The model under review builds one solid part; all positions refer to its coordinate system, in mm. Face numbers are marked on the shaded views. A direction names the side the tool comes from. Coordinates: 2 decimals unless noted, no trailing zeros. Loops run counter-clockwise (first coordinate to the right, second up) from the corner with the lowest first, then second, coordinate; pieces in that order, holes last. Notation, with made-up numbers: M 64,-6.5 L 92,-6.5 A12 cw 92,-1.5 Z; hole C 87.5,-28.75 d7. An arc over 180 degrees is marked long. One line per item, written item: value.
Autodesk Inventor part; units mm, degrees
ref_plane "aa2_XY" through (12.7, 0, 0) normal (0, 1, 0) x (1, 0, 0)
ref_plane "aa2_YZ" through (12.7, 0, 0) normal (1, 0, 0) x (0, 0, -1)
ref_plane "aa2_ZX" through (12.7, 0, 0) normal (0, 0, -1) x (0, 1, 0)
sketch "Sketch_1" plane through (0, 0, 0) normal (0, 0, 1) x (1, 0, 0)
  line L0 (12.7, 0) -> (0, 0)
  line L1 (0, 0) -> (0, 6.5151)
  line L2 (0, 6.5151) -> (0.762, 7.2771)
  line L3 (0.762, 7.2771) -> (2.7178, 7.2771)
  line L4 (2.7178, 7.2771) -> (3.3528, 6.6421)
  line L5 (3.3528, 6.6421) -> (3.9878, 6.6421)
  line L6 (3.9878, 6.6421) -> (3.9878, 7.747)
  line L7 (3.9878, 7.747) -> (11.938, 7.747)
  line L8 (11.938, 7.747) -> (12.7, 6.985)
  line L9 (12.7, 6.985) -> (12.7, 0)
  line L10 (12.7, 0) -> (0, 0)
revolve "Revolution1" add sketch "Sketch_1" angle 360 about axis through (12.7, 0, 0) along (1, 0, 0)
sketch "Sketch_2" plane through (12.7, 0, 0) normal (1, 0, 0) x (0, 0, -1)
  line L0 (-30.988, 12.573) -> (-30.988, -12.573)
  line L1 (-30.988, -12.573) -> (30.988, -12.573)
  line L2 (30.988, -12.573) -> (30.988, 12.573)
  line L3 (30.988, 12.573) -> (-30.988, 12.573)
  line L4 (-15.494, 6.2865) -> (-15.494, -6.2865)
  line L5 (-15.494, -6.2865) -> (15.494, -6.2865)
  line L6 (15.494, -6.2865) -> (15.494, 6.2865)
  line L7 (15.494, 6.2865) -> (-15.494, 6.2865)
extrude "Extrusion1" cut sketch "Sketch_2" against normal blind 4.699
sketch "Sketch3" plane through (0, 0, 0) normal (-1, 0, 0) x (0, 0, 1)
  point P0 (0, 0)
hole "Hole1" at (0, 0, 0) direction (1, 0, 0) diameter 9.525 depth 4.7752 countersink diameter 10.033 countersink angle 90
sketch "Sketch_5" plane through (0, 0, 0) normal (0, 0, 1) x (1, 0, 0)
  line L0 (12.7, 0) -> (-0.381, 0)
  line L1 (-0.381, 0) -> (-0.381, 1.9837)
  line L2 (-0.381, 1.9837) -> (11.8897, 1.9837)
  line L3 (11.8897, 1.9837) -> (12.319, 2.413)
  line L4 (12.319, 2.413) -> (12.319, 3.9624)
  line L5 (12.319, 3.9624) -> (12.7, 3.9624)
  line L6 (12.7, 3.9624) -> (12.7, 0)
  line L7 (12.7, 0) -> (-0.381, 0)
revolve "Revolution2" cut sketch "Sketch_5" angle 360 about axis through (12.7, 0, 0) along (1, 0, 0)
thread "Thread1"
sketch "Sketch_9" plane through (0, 0, 0) normal (0, 0, 1) x (1, 0, 0)
  line L0 (12.7, 0) -> (-12.7, 0)
  line L1 (3.2301, 7.6628) -> (4.2508, 6.6421)
  line L2 (4.2508, 6.6421) -> (4.5382, 6.6421)
  line L3 (4.5382, 6.6421) -> (3.4333, 7.747)
  line L4 (3.4333, 7.747) -> (3.2301, 7.747)
  line L5 (3.2301, 7.747) -> (3.2301, 7.6628)
revolve "Revolution3" add sketch "Sketch_9" angle 360 about axis through (12.7, 0, 0) along (1, 0, 0)
ref_plane "aa2_XY" through (12.7, 0, 0) normal (0, 1, 0) x (1, 0, 0)
ref_plane "aa2_YZ" through (12.7, 0, 0) normal (1, 0, 0) x (0, 0, -1)
ref_plane "aa2_ZX" through (12.7, 0, 0) normal (0, 0, -1) x (0, 1, 0)
ref_plane "m1_XY" through (12.7, 0, 0) normal (0, 1, 0) x (1, 0, 0)
ref_plane "m1_YZ" through (12.7, 0, 0) normal (1, 0, 0) x (0, 0, -1)
ref_plane "m1_ZX" through (12.7, 0, 0) normal (0, 0, -1) x (0, 1, 0)
ref_plane "m2_XY" through (8.001, 0, 0) normal (0, 1, 0) x (1, 0, 0)
ref_plane "m2_YZ" through (8.001, 0, 0) normal (1, 0, 0) x (0, 0, -1)
ref_plane "m2_ZX" through (8.001, 0, 0) normal (0, 0, -1) x (0, 1, 0)
ref_plane "n1_XY" through (12.7, 6.2865, 0) normal (1, 0, 0) x (0, 0, -1)
ref_plane "n1_YZ" through (12.7, 6.2865, 0) normal (0, 0, -1) x (0, 1, 0)
ref_plane "n1_ZX" through (12.7, 6.2865, 0) normal (0, 1, 0) x (1, 0, 0)
ref_plane "n2_XY" through (12.7, -6.2865, 0) normal (1, 0, 0) x (0, 0, -1)
ref_plane "n2_YZ" through (12.7, -6.2865, 0) normal (0, 0, -1) x (0, 1, 0)
ref_plane "n2_ZX" through (12.7, -6.2865, 0) normal (0, 1, 0) x (1, 0, 0)
ref_plane "rear_head_XY" through (2.7178, 0, 0) normal (1, 0, 0) x (0, 0, -1)
ref_plane "rear_head_YZ" through (2.7178, 0, 0) normal (0, 0, -1) x (0, 1, 0)
ref_plane "rear_head_ZX" through (2.7178, 0, 0) normal (0, 1, 0) x (1, 0, 0)
ref_plane "to_bushing_XY" through (0, 0, 0) normal (0, 0, 1) x (1, 0, 0)
ref_plane "to_bushing_YZ" through (0, 0, 0) normal (1, 0, 0) x (0, 1, 0)
ref_plane "to_bushing_ZX" through (0, 0, 0) normal (0, 1, 0) x (0, 0, 1)
ref_plane "to_mounting_bracket_xp_XY" through (12.7, 0, 0) normal (1, 0, 0) x (0, 0, -1)
ref_plane "to_mounting_bracket_xp_YZ" through (12.7, 0, 0) normal (0, 0, -1) x (0, 1, 0)
ref_plane "to_mounting_bracket_xp_ZX" through (12.7, 0, 0) normal (0, 1, 0) x (1, 0, 0)
ref_plane "to_pivot_bracket_XY" through (0, 0, 0) normal (0, 0, 1) x (1, 0, 0)
ref_plane "to_pivot_bracket_YZ" through (0, 0, 0) normal (1, 0, 0) x (0, 1, 0)
ref_plane "to_pivot_bracket_ZX" through (0, 0, 0) normal (0, 1, 0) x (0, 0, 1)
properties part number "D-14216rear_head"
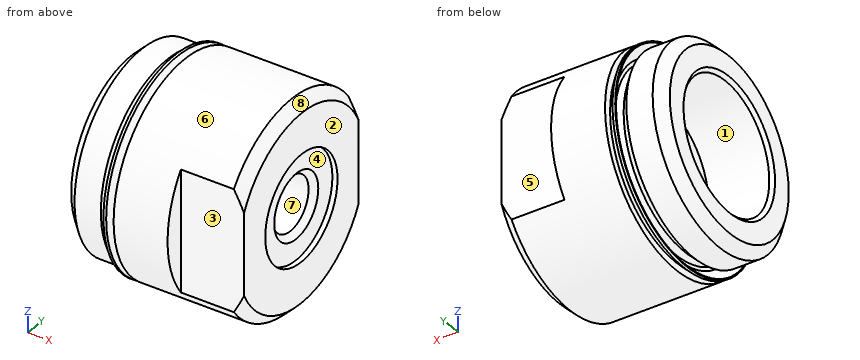
(1) Tool access review of the marked faces 1, 2, 3, 4 and 5: name each direction out of +Z, -Z, +X, -X, +Y, -Y from which nothing blocks a thin tool from reaching the whole face with its end or side.
Checks:
face 1: -X
face 2: +Z, -Z, +X, +Y, -Y
face 3: +Z, -Z, +X, -Y
face 4: +X
face 5: +Z, -Z, +X, +Y
(2) Add section B-B on x = 6. State the section outline as (y, z) points.
Checks:
outline: C 0,0 d15.49; hole C 0,0 d3.97
(3) Draft analysis for pull direction Z (two halves, no side actions). For the marked faces 6, 7 and 8, state which applies: pulls with the +Z half, pulls with the -Z half, needs draft (parallel to the pull), parting line crosses it, or undercut.
Checks:
face 6: parting line crosses it
face 7: undercut
face 8: pulls with the +Z half
(4) Add section A-A on x = 8.75. State the section outline as (y, z) points, then the cut area to 3 significant figures.
Checks:
outline: M -6.29,-4.53 A7.75 ccw 6.29,-4.53 L 6.29,4.53 A7.75 ccw -6.29,4.53 Z; hole C 0,0 d3.97
area: 158 mm^2
(5) To check wall thickness, follow L1, parallel to X at y = -3, z = 1.25; L2, parallel to X at y = -2.5, z = -4; L3, parallel to Y at x = 11.5, z = 0.25. State the ranges of each line that lie inside material, in increasing order. Write a range as [from, to].
Checks:
L1: [4.78, 12.32]
L2: [4.78, 12.7]
L3: [-6.29, -1.97], [1.97, 6.29]
(6) Add section C-C on x = 3. State the section outline as (y, z) points (1 decimal).
Checks:
outline: C 0,0 d14; hole C 0,0 d9.5
(7) Insertion check: pin 1 Ø4.5 at (y, z) = (0, 0) entering from +X; pin 2 Ø0.7 at (y, z) = (-7, 2) entering from +X; pin 3 Ø1.5 at (y, z) = (3, -1) entering from -X. Each pin has a flat end and moves straight along its axis. Give the tip position at first contact, or say it passes through.
Checks:
pin 1: x = 12.16
pin 2: x = 8
pin 3: x = 4.78
